Source: CAD feature listing. Evaluate the final solid. Frame: model axes, mm. Coordinates: 2 decimals unless noted, no trailing zeros. Write each loop counter-clockwise with the first axis right and the second up, starting at its lowest first coordinate (ties: lowest second). Pieces come first, ordered by that corner, then holes. Notation, with made-up numbers: M 43.5,9 L 75.5,9 A28 cw 75.5,36 Z; hole C 43.5,-18 d5. An arc over 180 degrees is marked long. One line per item, written item: value. Start each with the question number.
Item 1: Cut plane A-A, the plane z = 0. Output: boundary loops of the cut face in (x, y), then the cut area to 3 significant figures.
Item 2: Cut plane B-B, the plane x = 20. Output: boundary loops of the cut face in (y, z), then the cut area to 3 significant figures.
Item 3: Cut plane C-C, the plane y = 7.5. Output: boundary loops of the cut face in (x, z).
Item 4: Ray query, L1, parallel to Y at x = -20, z = -1.5; L2, parallel to Y at x = -21.5, z = 5.5; L3, parallel to Z at x = -5, y = 15. Return the intervals inside material, ascending. Write a range as from..to.
Item 5: Mould query, pull axis Y, two halves, no side actions, for faces 1 (the cylindrical face through (21.038, 16.004, -0.227)), 2 (the flat face through (-27, 0, 0)), 3 (the flat face through (-6.4, 25.25, 0.2)). Classes: released by +Y, released by -Y, zero draft, split by the parting line, or undercut.
Item 6: Pin query (flat end, axial travel): P1, Ø9.5, axis at x = 0, z = 0, coming from the -Y side. Return the tip coordinate at first contact, or that it passes through.
Item 7: Cut plane D-D, the plane z = 9.5. Output: boundary loops of the cut face in (x, y), then the cut area to 3 significant figures.
```python
from build123d import *

# Parameters (mm, degrees)
SKETCH_W     = 54
SKETCH_H     = 50.5
SKETCH_R     = 2.25
PAD_DEPTH    = 16.25
SKETCH001_R  = 6
POCKET_DEPTH = 50.5


with BuildPart() as part:
    # Sketch → Pad (new body, symmetric)
    with BuildSketch(Plane.XY):
        Rectangle(SKETCH_W, SKETCH_H)
        with Locations((-20, 18)):
            Circle(SKETCH_R, mode=Mode.SUBTRACT)
        with Locations((-20, -18)):
            Circle(SKETCH_R, mode=Mode.SUBTRACT)
        with Locations((20, 18)):
            Circle(SKETCH_R, mode=Mode.SUBTRACT)
        with Locations((20, -18)):
            Circle(SKETCH_R, mode=Mode.SUBTRACT)
    extrude(amount=PAD_DEPTH, both=True)

    # Sketch001 → Pocket (cut)
    with BuildSketch(Plane.XZ.offset(25.25)):
        Circle(SKETCH001_R)
    extrude(amount=-POCKET_DEPTH, mode=Mode.SUBTRACT)


solid = part.part
```
From the geometry:
1. outline: M -27,-25.25 L -6,-25.25 L -6,25.25 L -27,25.25 Z; M 6,-25.25 L 27,-25.25 L 27,25.25 L 6,25.25 Z; hole C -20,-18 d4.5; hole C -20,18 d4.5; hole C 20,-18 d4.5; hole C 20,18 d4.5
1. area: 2,060 mm²
2. outline: M -25.25,-16.25 L -20.25,-16.25 L -20.25,16.25 L -25.25,16.25 Z; M -15.75,-16.25 L 15.75,-16.25 L 15.75,16.25 L -15.75,16.25 Z; M 20.25,-16.25 L 25.25,-16.25 L 25.25,16.25 L 20.25,16.25 Z
2. area: 1,350 mm²
3. outline: M -27,-16.25 L 27,-16.25 L 27,16.25 L -27,16.25 Z; hole C 0,0 d12
4. L1: y = -25.25..-20.25, -15.75..15.75, 20.25..25.25
4. L2: y = -25.25..-19.68, -16.32..16.32, 19.68..25.25
4. L3: z = -16.25..-3.32, 3.32..16.25
5. face 1: undercut
5. face 2: zero draft
5. face 3: released by +Y
6. P1: passes through
7. outline: M -27,-25.25 L 27,-25.25 L 27,25.25 L -27,25.25 Z; hole C -20,-18 d4.5; hole C -20,18 d4.5; hole C 20,-18 d4.5; hole C 20,18 d4.5
7. area: 2,660 mm²
